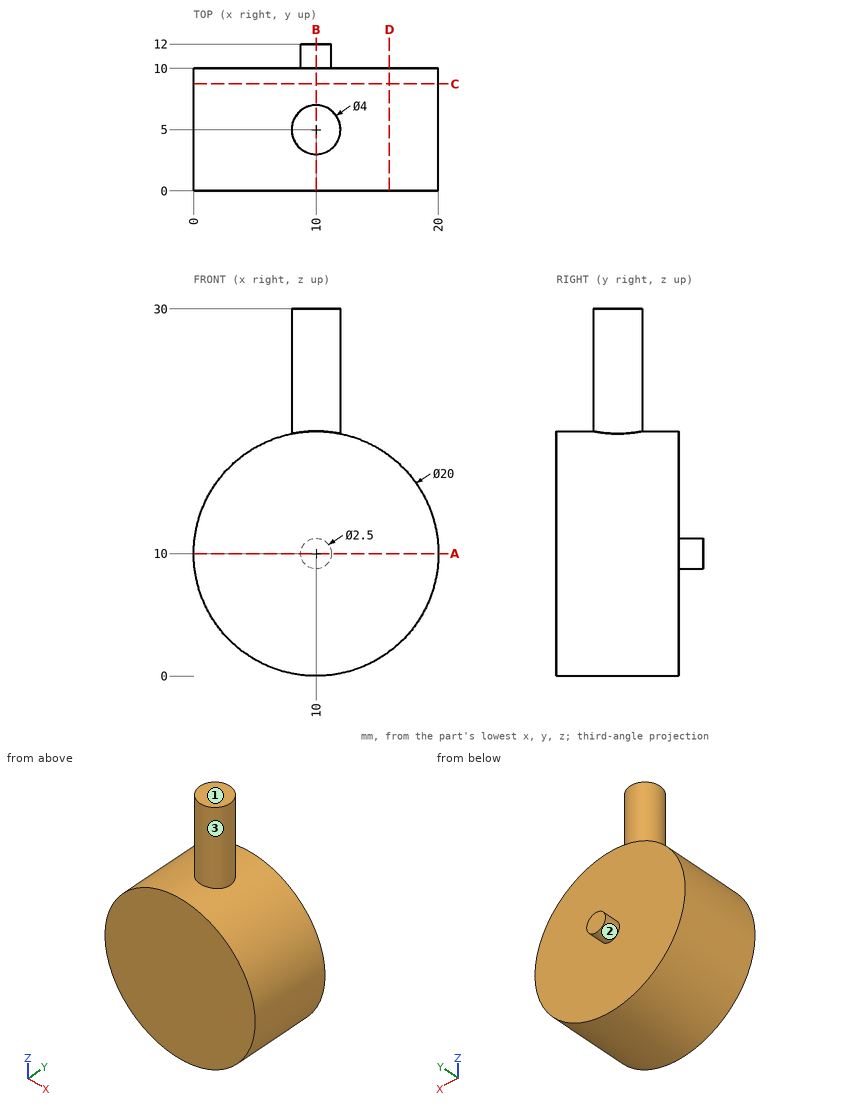
Verification items for this drawing (mm, ordinates from the low corner). A direction names the side the tool comes from. Round coordinates to 2 decimals unless told otherwise and drop trailing zeros. Loops run counter-clockwise (first coordinate to the right, second up) from the corner with the lowest first, then second, coordinate; pieces in that order, holes last. Notation, with made-up numbers: (6, -23.5) -> (17, -23.5) arc R34 ccw to (17, 13.5) -> close; hole circle Ø2 at (46, 26.25). An arc over 180 degrees is marked (long way). Write item = value, one per line. Start each with the question number.
1) Gauge pin test, flat ends, axial feed: pin 1 Ø4 at (y, z) = (8, 20.5) entering from -X; pin 2 Ø1 at (x, y) = (4, 7) entering from +Z; pin 3 Ø12 at (x, z) = (9.5, 20.5) entering from -Y; pin 4 Ø1 at (x, y) = (3.5, 6) entering from -Z. Record the tip position at first contact, or that the pin passes through.
2) Sectioned sample at A-A, the plane z = 10. Record the cut outline in (x, y), plus the area to 3 significant figures.
3) Thickness scan on probe 1 along Y at (x, z) = (7.5, 5.5); probe 2 along X at (y, z) = (1, 14); probe 3 along X at (y, z) = (5.5, 28.5). Record the ranges inside material, lowest first.
4) Sectioned sample at D-D, the plane x = 16. Record the cut outline in (y, z), plus the area to 3 significant figures.
5) Sectioned sample at B-B, the plane x = 10. Record the cut outline in (y, z), plus the area to 3 significant figures.
6) Sectioned sample at C-C, the plane y = 8.75. Record the cut outline in (x, z), plus the area to 3 significant figures.
7) Set-up check for the marked faces 1, 2 and 3: record each of +Z, -Z, +X, -X, +Y, -Y from which the full face is reachable in a straight line by a thin tool's end or side.
Results are:
q1.pin_1 = 4.73
q1.pin_2 = 18.35
q1.pin_3 = 0
q1.pin_4 = 2
q2.outline = (0, 0) -> (20, 0) -> (20, 10) -> (11.25, 10) -> (11.25, 12) -> (8.75, 12) -> (8.75, 10) -> (0, 10) -> close
q2.area = 205 mm^2
q3.probe_1 = 0 to 10
q3.probe_2 = 0.83 to 19.17
q3.probe_3 = 8.06 to 11.94
q4.outline = (0, 2) -> (10, 2) -> (10, 18) -> (0, 18) -> close
q4.area = 160 mm^2
q5.outline = (0, 0) -> (10, 0) -> (10, 8.75) -> (12, 8.75) -> (12, 11.25) -> (10, 11.25) -> (10, 20) -> (7, 20) -> (7, 30) -> (3, 30) -> (3, 20) -> (0, 20) -> close
q5.area = 245 mm^2
q6.outline = circle Ø20 at (10, 10)
q6.area = 314 mm^2
q7.face_1 = +Z, +X, -X, +Y, -Y
q7.face_2 = +Y
q7.face_3 = +Z
